Build history of the part. All positions in model axes, mm. Coordinates: 2 decimals unless noted, no trailing zeros. Write each loop counter-clockwise with the first axis right and the second up, starting at its lowest first coordinate (ties: lowest second). Pieces come first, ordered by that corner, then holes. Notation, with made-up numbers: M 44,49 L 87,49 A29 ccw 87,79 Z; hole C 78.25,-16 d6. An arc over 180 degrees is marked long. Use CSV: the item, a comma, the result in double quotes. Start each with the question number.
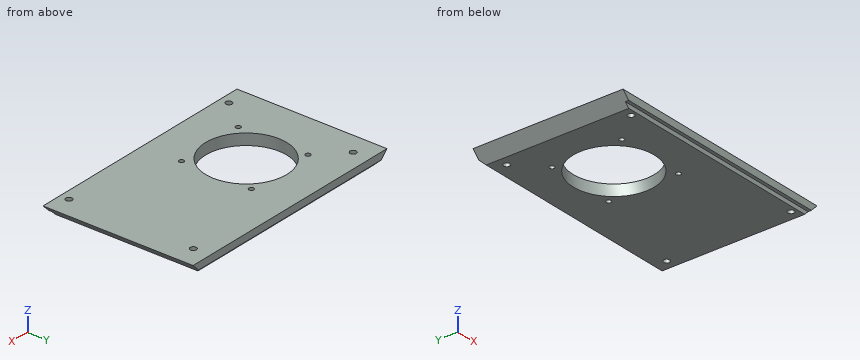
```python
from build123d import *

# Parameters (mm, degrees)
SKETCH1_W           = 171
SKETCH1_H           = 110
SKETCH1_R           = 2.25
BOSS_EXTRUDE1_DEPTH = 5
SKETCH2_W           = 171
SKETCH2_H           = 105
SKETCH2_R           = 2.25
BOSS_EXTRUDE2_DEPTH = 3
CHAMFER1_SIZE       = 8
CHAMFER3_SIZE       = 3
SKETCH3_W           = 7.071067812
SKETCH3_H           = 2.6
CUT_EXTRUDE1_DEPTH  = 232.587308883
SKETCH4_R           = 29
SKETCH4_R_2         = 1.75
CUT_EXTRUDE2_DEPTH  = 204.482185952


with BuildPart() as part:
    # Sketch1 → Boss-Extrude1 (new body)
    with BuildSketch(Plane.XY):
        with Locations((85.5, 55)):
            Rectangle(SKETCH1_W, SKETCH1_H)
        with Locations((15, 9)):
            Circle(SKETCH1_R, mode=Mode.SUBTRACT)
        with Locations(Location((156, 9, 0), (0, 0, 180))):
            Circle(SKETCH1_R, mode=Mode.SUBTRACT)
        with Locations((15, 98)):
            Circle(SKETCH1_R, mode=Mode.SUBTRACT)
        with Locations(Location((156, 98, 0), (0, 0, 180))):
            Circle(SKETCH1_R, mode=Mode.SUBTRACT)
    extrude(amount=-BOSS_EXTRUDE1_DEPTH)

    # Sketch2 → Boss-Extrude2 (add)
    with BuildSketch(Plane(origin=(0, 0, -5), x_dir=(-1, 0, 0), z_dir=(0, 0, -1))):
        with Locations((-85.5, 57.5)):
            Rectangle(SKETCH2_W, SKETCH2_H)
        with Locations(Location((-15, 9, 0), (0, 0, 180))):
            Circle(SKETCH2_R, mode=Mode.SUBTRACT)
        with Locations((-156, 9)):
            Circle(SKETCH2_R, mode=Mode.SUBTRACT)
        with Locations(Location((-15, 98, 0), (0, 0, 180))):
            Circle(SKETCH2_R, mode=Mode.SUBTRACT)
        with Locations((-156, 98)):
            Circle(SKETCH2_R, mode=Mode.SUBTRACT)
    extrude(amount=BOSS_EXTRUDE2_DEPTH)

    # Chamfer1
    # the kernel refuses this chamfer: 8 mm, written as the material it takes off along each edge
    with BuildSketch(Plane(origin=(171, -15.573463904, -8), x_dir=(-0.9996219169112968, 0, -0.027495876610586296), z_dir=(0, 1, 0)), Plane(origin=(0, 130.573463904, -8), x_dir=(0.9996219169112968, 0, -0.027495876610586275), z_dir=(0, -1, 0))) as chamfer1_piece_1:
        Polygon((CHAMFER1_SIZE * 0.999621916911, CHAMFER1_SIZE * 0.0274958766106), (-CHAMFER1_SIZE * 0.0274958766106, CHAMFER1_SIZE * 0.999621916911), (0, 0), align=None)
    extrude(amount=146.146927807, mode=Mode.SUBTRACT)

    # Chamfer3
    chamfer3_edges = [part.edges().sort_by_distance(p)[0] for p in [
        (85.5, 110, -8),
    ]]
    chamfer(chamfer3_edges, length=CHAMFER3_SIZE)

    # Sketch3 → Cut-Extrude1 (cut, through all, along a direction that is not the sketch's normal)
    with BuildSketch(Plane(origin=(85.5, 0, -85.5), x_dir=(-0.7071067811865452, 0, -0.7071067811865498), z_dir=(0.7071067811865498, 0, -0.7071067811865452))):
        with Locations((-117.379725677, 1.3)):
            Rectangle(SKETCH3_W, SKETCH3_H)
    extrude(amount=-CUT_EXTRUDE1_DEPTH, dir=(1, 0, 0), mode=Mode.SUBTRACT)

    # Sketch4 → Cut-Extrude2 (cut, through all)
    with BuildSketch(Plane.XY):
        with Locations((58, 56.3)):
            Circle(SKETCH4_R)
        with Locations((33, 80.3)):
            Circle(SKETCH4_R_2)
        with Locations((83, 80.3)):
            Circle(SKETCH4_R_2)
        with Locations((83, 30.3)):
            Circle(SKETCH4_R_2)
        with Locations((33, 30.3)):
            Circle(SKETCH4_R_2)
    extrude(amount=-CUT_EXTRUDE2_DEPTH, mode=Mode.SUBTRACT)


solid = part.part
```
1. Slice it at C-C (y = 56.3). List the corners of the cut face in (x, z).
2. Drill centre lines: line 1 along Y through (x, z) = (156, -2.4); line 2 along Y through (x, z) = (33, -2.75); line 3 along X through (y, z) = (99, -0.75). Where is each one in solid material? Low to high. Write a range as from..to.
3. Slice it at B-B (z = -2). Count the separate pieces of the cut face and the enclosed holes in it, and give its area (3 significant figures).
4. Flat gauge pins, fed straight in: pin 1 (5 mm diameter, centred on x = 15, y = 98, fed in from -Z); pin 2 (1.2 mm diameter, centred on x = 122.5, y = 3.5, fed in from -Z); pin 3 (3 mm diameter, centred on y = 22, z = -2, fed in from -X); pin 4 (2 mm diameter, centred on y = 82, z = -6.5, fed in from +X). Where does each tip first touch, or does it go through?
5. Slice it at D-D (x = 83). List the corners of the cut face in (y, z), and give its area (3 significant figures).
6. Slice it at A-A (x = 15). List the corners of the cut face in (y, z), and give its area (4 significant figures).
Established:
1,outline,"M 0,0 L 8,-8 L 29,-8 L 29,0 Z; M 87,-8 L 163,-8 L 171,0 L 87,0 Z"
2,line 1,"y = 2.6..6.75, 11.25..95.75, 100.25..110"
2,line 2,"y = 2.6..28.55, 32.05..41.6, 71..78.55, 82.05..110"
2,line 3,"x = 0.75..12.98, 17.02..153.98, 158.02..170.25"
3,separate pieces,"1"
3,enclosed holes,"9"
3,area,"15,200 mm2"
4,pin 1,"stops at z = -8"
4,pin 2,"stops at z = -5"
4,pin 3,"stops at x = 0.5"
4,pin 4,"stops at x = 165.5"
5,outline,"M 2.6,-5 L 5,-5 L 5,-8 L 28.55,-8 L 28.55,0 L 2.6,0 Z; M 32.05,-8 L 41.6,-8 L 41.6,0 L 32.05,0 Z; M 71,-8 L 78.55,-8 L 78.55,0 L 71,0 Z; M 82.05,-8 L 107,-8 L 110,-5 L 110,0 L 82.05,0 Z"
5,area,"556 mm2"
6,outline,"M 2.6,-5 L 5,-5 L 5,-8 L 6.75,-8 L 6.75,0 L 2.6,0 Z; M 11.25,-8 L 95.75,-8 L 95.75,0 L 11.25,0 Z; M 100.25,-8 L 107,-8 L 110,-5 L 110,0 L 100.25,0 Z"
6,area,"775.5 mm2"
